Input: part model. Units: mm. Frame: model coordinates. Face numbers are marked on the shaded views. Coordinates: 2 decimals unless noted, no trailing zeros. Order: outer loops, then holes, each group sorted by start corner. A loop starts at its lowest first (then second) coordinate and runs counter-clockwise, first axis right, second up. Notation, with made-up numbers: (35.25, 53.25) - (68.25, 53.25) arc R11 ccw to (68.25, 62.25) - close; hole circle Ø2 at (-19.75, 65). An arc over 180 degrees is marked (long way). Answer as CSV lines item,"result". Start each with the question number.
Item 1: First-contact query: pin 1 (3 mm diameter, centred on x = 0, z = 7.5, fed in from -Y); pin 2 (1 mm diameter, centred on y = -0.5, z = 3, fed in from -X). Flat tips, straight axial feed; report the tip coordinate or a pass-through.
Item 2: Draft query along Z for the marked faces 1, 2, 3 and 4. Return one class per face: +Z half, -Z half, draft (parallel to the pull), parting line (faces both ways), or undercut.
Item 3: Section C-C (z = 2.5). Output: boundary loops of the cut face in (x, y), and give its area (3 significant figures).
Item 4: Section D-D (z = 1.5). Output: boundary loops of the cut face in (x, y).
Item 5: Section B-B (y = 0). Output: boundary loops of the cut face in (x, z).
Item 6: Section A-A (x = 0.1). Output: boundary loops of the cut face in (y, z).
Item 7: Material intervals for line 1 along Z through (x, y) = (1.2, 1.25); line 2 along Y through (x, z) = (-0.45, 2.5); line 3 along Z through (x, y) = (0, 0.25), sorted ascending.
from build123d import *

# Parameters (mm, degrees)
SKETCH1_W           = 5
SKETCH1_H           = 5
BOSS_EXTRUDE1_DEPTH = 10
SKETCH4_R           = 1.6
CUT_EXTRUDE3_DEPTH  = 4.5
SKETCH5_R           = 1.6
CUT_EXTRUDE4_DEPTH  = 4.5
CHAMFER1_SIZE       = 0.5
CHAMFER4_SIZE       = 0.4


with BuildPart() as part:
    # Sketch1 → Boss-Extrude1 (new body)
    with BuildSketch(Plane.XY):
        Rectangle(SKETCH1_W, SKETCH1_H)
    extrude(amount=BOSS_EXTRUDE1_DEPTH)

    # Sketch4 → Cut-Extrude3 (cut)
    with BuildSketch(Plane.XZ.offset(2.5)):
        with Locations((0, 7.5)):
            Circle(SKETCH4_R)
    extrude(amount=-CUT_EXTRUDE3_DEPTH, mode=Mode.SUBTRACT)

    # Sketch5 → Cut-Extrude4 (cut)
    with BuildSketch(Plane.ZY.offset(2.5)):
        with Locations((2.5, 0)):
            Circle(SKETCH5_R)
    extrude(amount=-CUT_EXTRUDE4_DEPTH, mode=Mode.SUBTRACT)

    # Chamfer1
    chamfer1_edges = [part.edges().sort_by_distance(p)[0] for p in [
        (-2.5, -2.5, 5),
    ]]
    chamfer(chamfer1_edges, length=CHAMFER1_SIZE)

    # Chamfer4
    chamfer4_edges = [part.edges().sort_by_distance(p)[0] for p in [
        (0.25, -2.5, 0),
        (-2.25, -2.25, 0),
        (-2.5, 0.25, 0),
    ]]
    chamfer(chamfer4_edges, length=CHAMFER4_SIZE)


solid = part.part
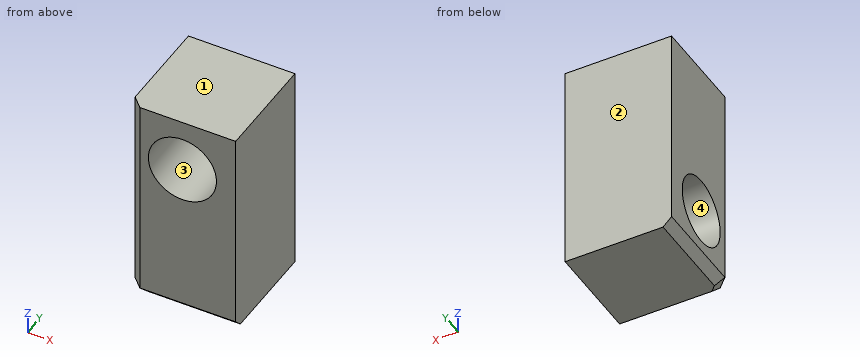
Determined:
1,pin 1,"stops at y = 2"
1,pin 2,"stops at x = 2"
2,face 1,"+Z half"
2,face 2,"draft"
2,face 3,"undercut"
2,face 4,"undercut"
3,outline,"(-2.5, -2) - (-2, -2.5) - (2.5, -2.5) - (2.5, 2.5) - (-2.5, 2.5) - (-2.5, 1.6) - (2, 1.6) - (2, -1.6) - (-2.5, -1.6) - close"
3,area,"10.5 mm^2"
4,outline,"(-2.5, -2) - (-2, -2.5) - (2.5, -2.5) - (2.5, 2.5) - (-2.5, 2.5) - (-2.5, 1.25) - (2, 1.25) - (2, -1.25) - (-2.5, -1.25) - close"
5,outline,"(-2.5, 0.4) - (-2.1, 0) - (2.5, 0) - (2.5, 10) - (-2.5, 10) - (-2.5, 4.1) - (2, 4.1) - (2, 0.9) - (-2.5, 0.9) - close; hole circle Ø3.2 at (0, 7.5)"
6,outline,"(-2.5, 0.4) - (-2.1, 0) - (2.5, 0) - (2.5, 10) - (-2.5, 10) - (-2.5, 9.1) - (2, 9.1) - (2, 5.9) - (-2.5, 5.9) - close; hole circle Ø3.2 at (0, 2.5)"
7,line 1,"z = 0 to 1.5, 3.5 to 6.44, 8.56 to 10"
7,line 2,"y = -2.5 to -1.6, 1.6 to 2.5"
7,line 3,"z = 0 to 0.92, 4.08 to 5.9, 9.1 to 10"
